Part model, mm, in its own coordinate system. A direction names the side the tool comes from. Give positions to 0.01 mm unless a question says otherwise; leave off trailing zeros. Loops run counter-clockwise (first coordinate to the right, second up) from the corner with the lowest first, then second, coordinate; pieces in that order, holes last. Notation, with made-up numbers: M 49.5,52.25 L 70.5,52.25 A22 ccw 70.5,58.25 Z; hole C 85.25,-1 d2. An arc over 180 degrees is marked long. Put each result on its own line as item: value. Start each with the question number.
```python
from build123d import *

# Parameters (mm, degrees)
F0_R     = 4
F0_R_2   = 1.875
F1_DEPTH = 10
F2_R     = 4
F3_DEPTH = 2
F4_R     = 0.75
F5_DEPTH = 1.5
F6_SIZE  = 0.25
F7_R     = 4
F8_DEPTH = 10
F9_R     = 0.25
F10_R    = 0.25


with BuildPart() as f1:
    # F0 (on Top) → F1 (new body)
    with BuildSketch(Plane.XY):
        Circle(F0_R)
        Circle(F0_R_2, mode=Mode.SUBTRACT)
    extrude(amount=F1_DEPTH)

    # F2 (on face) → F3 (join)
    with BuildSketch(Plane.XY.offset(10)):
        Circle(F2_R)
    extrude(amount=F3_DEPTH)

    # F4 (on face) → F5 (join)
    with BuildSketch(Plane.XY.offset(12)):
        Circle(F4_R)
    extrude(amount=F5_DEPTH)

    # F6
    f6_edges = [f1.edges().sort_by_distance(p)[0] for p in [
        (-0.75, 0, 13.5),
    ]]
    chamfer(f6_edges, length=F6_SIZE)

    # F7 (on face) → F8 (join)
    with BuildSketch(Plane.XY.offset(12)):
        Circle(F7_R)
        Polygon((-0.447693, -2.290151), (-2.290151, 0.447693), (0.447693, 2.290151), (2.290151, -0.447693), align=None, mode=Mode.SUBTRACT)
    extrude(amount=F8_DEPTH)

    # F9
    f9_edges = [f1.edges().sort_by_distance(p)[0] for p in [
        (-4, 0, 22),
    ]]
    fillet(f9_edges, radius=F9_R)

    # F10
    f10_edges = [f1.edges().sort_by_distance(p)[0] for p in [
        (-4, 0, 0),
    ]]
    fillet(f10_edges, radius=F10_R)


solid = f1.part
```
1) Band-saw the part on D-D on z = 11. Give the cut face in (x, y).
2) Which spindle directions (+Z, -Z, +X, -X, +Y, -Y) get a long thin tool onto all of the face, cutting with end or side? Do faces 4 (the flat face through (1, -2, 22)), 5 (the flat face through (-0.94, 1.356, 16.93)), 6 (the flat face through (0, 0, 10)). Say none if no direction does.
3) Mould opens along Y. For faces 1 (the flat face through (1, 2, 0)), 2 (the flat face through (-1.356, -0.94, 16.93)), 3 (the cylindrical face through (-0.867, -3.905, 10.849)) say: +Y half, -Y half, draft (parallel to the pull), parting line (faces both ways), or undercut.
4) Wall check: L1, parallel to Y at x = 0, z = 7.25 (3 decimals); L2, parallel to X at y = -0.5, z = 2.75; L3, parallel to Z at x = -0.5, y = 1.25. Give the ranges that are in metal, low to high.
5) Band-saw the part on B-B on y = 0. Give the cut face in (x, z) (3 decimals).
6) Band-saw the part on A-A on z = 16.75. Give the cut face in (x, y).
7) Pin check, flat tips, straight feed: pin 1 Ø1.5 at (y, z) = (2, 15.5) entering from +X; pin 2 Ø4 at (x, z) = (-3, 18) entering from -Y; pin 3 Ø1 at (x, z) = (-2.5, 19.5) entering from -Y. Stop position of each tip, or through.
Evaluation:
1. outline: C 0,0 d8
2. face 4: +Z, +X, -X, +Y, -Y
2. face 5: +Z
2. face 6: -Z
3. face 1: draft
3. face 2: undercut
3. face 3: parting line
4. L1: -4 to -1.875, 1.875 to 4
4. L2: -3.97 to -1.81, 1.81 to 3.97
4. L3: 10 to 12
5. outline: M -4,0.25 A0.25 ccw -3.75,0 L -1.875,0 L -1.875,10 L 1.875,10 L 1.875,0 L 3.75,0 A0.25 ccw 4,0.25 L 4,21.75 A0.25 ccw 3.75,22 L 1.989,22 L 1.989,12 L 0.75,12 L 0.75,13.25 L 0.5,13.5 L -0.5,13.5 L -0.75,13.25 L -0.75,12 L -1.989,12 L -1.989,22 L -3.75,22 A0.25 ccw -4,21.75 Z
6. outline: C 0,0 d8; hole M -2.29,0.45 L -0.45,-2.29 L 2.29,-0.45 L 0.45,2.29 Z
7. pin 1: x = 3.8
7. pin 2: y = -3.87
7. pin 3: y = -3.46
